from build123d import *

# Parameters (mm, degrees)
BASE_FLANGE1_DEPTH      = 10
BASE_FLANGE1_DEPTH_BACK = 5
CUT_EXTRUDE1_DEPTH      = 10
CUT_EXTRUDE2_DEPTH      = 10


# Sheet-metal steps are written as plain solids
with BuildPart() as part:
    # Sketch1 → Base-Flange1 (new, two sides: drawn at the far end of the back side and taken through both)
    with BuildSketch(Plane.XY.offset(-BASE_FLANGE1_DEPTH_BACK)):
        with BuildLine():
            Line((0, 0), (0, -42.4))
            ThreePointArc((0, -42.4), (0.761522369, -44.238477631), (2.6, -45))
            Line((2.6, -45), (45, -45))
            Line((45, -45), (45, -47))
            Line((45, -47), (2.6, -47))
            ThreePointArc((2.6, -47), (-0.652691193, -45.652691193), (-2, -42.4))
            Line((-2, -42.4), (-2, 0))
            Line((-2, 0), (0, 0))
        make_face()
    extrude(amount=BASE_FLANGE1_DEPTH + BASE_FLANGE1_DEPTH_BACK)

    # Sketch6 → Cut-Extrude1 (cut)
    with BuildSketch(Plane(origin=(0, 0, 0), x_dir=(0, 0, -1), z_dir=(1, 0, 0))):
        with BuildLine():
            Line((-1, -5), (-1, -30))
            ThreePointArc((-1, -30), (-2.5, -31.5), (-4, -30))
            Line((-4, -30), (-4, -5))
            ThreePointArc((-4, -5), (-2.5, -3.5), (-1, -5))
        make_face()
    extrude(amount=-CUT_EXTRUDE1_DEPTH, mode=Mode.SUBTRACT)

    # Sketch7 → Cut-Extrude2 (cut)
    with BuildSketch(Plane(origin=(0, -45, 0), x_dir=(1, 0, 0), z_dir=(0, 1, 0))):
        with BuildLine():
            Line((40, -4), (15, -4))
            ThreePointArc((15, -4), (13.5, -2.5), (15, -1))
            Line((15, -1), (40, -1))
            ThreePointArc((40, -1), (41.5, -2.5), (40, -4))
        make_face()
    extrude(amount=-CUT_EXTRUDE2_DEPTH, mode=Mode.SUBTRACT)


solid = part.part
Work out the finished part from the listing and answer in its coordinate system (mm). A direction names the side the tool comes from. Give positions to 0.01 mm unless a question says otherwise; leave off trailing zeros. Order: outer loops, then holes, each group sorted by start corner. A loop starts at its lowest first (then second) coordinate and runs counter-clockwise, first axis right, second up. Notation, with made-up numbers: (-0.75, 69.5) -> (29.25, 69.5) arc R12 ccw to (29.25, 88.5) -> close; hole circle Ø7 at (12.5, 34). An arc over 180 degrees is marked (long way). One line per item, written item: value.
Item 1: Find section C-C, the plane y = -10.5. Give the vertices of the cut face in (x, z).
Answer sheet:
outline: (-2, -5) -> (0, -5) -> (0, 1) -> (-2, 1) -> close; (-2, 4) -> (0, 4) -> (0, 10) -> (-2, 10) -> close
Item 2: Find section A-A, the plane z = 2.5. Give the vertices of the cut face in (x, y).
Answer sheet:
outline: (-2, -42.4) arc R4.6 ccw to (2.6, -47) -> (13.5, -47) -> (13.5, -45) -> (2.6, -45) arc R2.6 cw to (0, -42.4) -> (0, -31.5) -> (-2, -31.5) -> close; (-2, -3.5) -> (0, -3.5) -> (0, 0) -> (-2, 0) -> close; (41.5, -47) -> (45, -47) -> (45, -45) -> (41.5, -45) -> close
Item 3: Flat-ended cylindrical pins translate along their axes: P1, Ø2, axis at x = 24, z = 0, coming from the +Y side; P2, Ø6, axis at y = -26, z = 8.5, coming from the +X side; P3, Ø12, axis at x = 34.5, y = -38, coming from the -Z side. Find the tip coordinate at first contact, or state that the pin passes through.
Answer sheet:
P1: y = -45
P2: x = 0
P3: through
Item 4: Find section B-B, the plane x = 36.5. Give the vertices of the cut face in (y, z), plus the area to 3 significant figures.
Answer sheet:
outline: (-47, -5) -> (-45, -5) -> (-45, 1) -> (-47, 1) -> close; (-47, 4) -> (-45, 4) -> (-45, 10) -> (-47, 10) -> close
area: 24.0 mm²
Item 5: A tool of negligible diameter and unlimited length cuts with its end or side. For faces 1 (the flat face through (23.5, -45, 0.7)), 2 (the cylindrical face through (41.5, -46, 2.5)), 3 (the cylindrical face through (-1, -31.5, 2.5)), from which of +Z, -Z, +X, -X, +Y, -Y can it reach the whole face along a straight path? Write none if from no direction.
Answer sheet:
face 1: +Z, -Z, +X, +Y
face 2: +Y, -Y
face 3: +X, -X
Item 6: Determine the mould class of faces 4 (the flat face through (27, -46, 1)), 5 (the cylindrical face through (0.741, -44.218, 2.395)), 6 (the flat face through (11, -46, -5)) for opening direction Z: released by +Z, released by -Z, zero draft, split by the parting line, or undercut.
Answer sheet:
face 4: undercut
face 5: zero draft
face 6: released by -Z
Item 7: Straight lines are drawn through the part: probe 1 along X at (y, z) = (-33.5, -3.5); probe 2 along Y at (x, z) = (27.5, 0.5). For each, find the intervals that lie inside material, in ascending order.
Answer sheet:
probe 1: -2 to 0
probe 2: -47 to -45
Item 8: Find section D-D, the plane z = -1. Give the vertices of the cut face in (x, y).
Answer sheet:
outline: (-2, -42.4) arc R4.6 ccw to (2.6, -47) -> (45, -47) -> (45, -45) -> (2.6, -45) arc R2.6 cw to (0, -42.4) -> (0, 0) -> (-2, 0) -> close
